Build history of the part. All positions in model axes, mm. A direction names the side the tool comes from. Give positions to 0.01 mm unless a question says otherwise; leave off trailing zeros. Order: outer loops, then holes, each group sorted by start corner. A loop starts at its lowest first (then second) coordinate and runs counter-clockwise, first axis right, second up. Notation, with made-up numbers: (59.25, 11.25) - (106.25, 11.25) arc R19 cw to (106.25, 41.25) - close; hole circle Ø10 at (23.5, -28). An arc over 180 degrees is marked (long way). Use a Markdown table: item, result. Add a question column.
(1) Flat gauge pins, fed straight in: pin 1 (2 mm diameter, centred on x = 8, z = 14, fed in from -Y); pin 2 (1.1 mm diameter, centred on y = -8.5, z = 4.5, fed in from +X); pin 3 (8 mm diameter, centred on x = 2, y = 4.5, fed in from +Z). Where does each tip first touch, or does it go through?
(2) Slice it at C-C (z = 12.5). Write the cut outline in (x, y).
(3) Slice it at B-B (y = 12). Write the cut outline in (x, z).
(4) Slice it at D-D (z = 21.5). Write the cut outline in (x, y).
(5) Wall check: line 1 (X direction, y = 4, z = 12.25); line 2 (Y direction, x = 0, z = 16.5); line 3 (Y direction, x = 0, z = 23.2). Give the ranges that are in metal, low to high.
(6) Which spindle directions (+Z, -Z, +X, -X, +Y, -Y) get a long thin tool onto all of the face, cutting with end or side? Do faces 5 (the face through (-2.17, -9.76, 19.96)), 6 (the face through (4.38, -8.43, 23.25)), 7 (the face through (6.3, -9, 7)), 8 (the face through (-8.8, -4.2, 7.4)). Say none if no direction does.
(7) Slice it at A-A (x = 0). Write the cut outline in (y, z).
(8) Mould opens along Z. For faces 1 (the face through (0, 13.5, 7)), 2 (the face through (0, 7, 15)), 3 (the face through (0, 13, 17)), 4 (the face through (9, -4, 23)) say: +Z half, -Z half, draft (parallel to the pull), parting line (faces both ways), or undercut.
from build123d import *

# Parameters (mm, degrees)
F1_DEPTH = 15
F3_DEPTH = 2
F4_R     = 11.5
F4_R_2   = 10
F5_DEPTH = 7
F6_R     = 11.5
F6_R_2   = 9.5
F7_DEPTH = 1
F8_R     = 0.5


with BuildPart() as f1:
    # F0 (on Top) → F1 (new body)
    with BuildSketch(Plane.XY):
        with BuildLine():
            ThreePointArc((-6.3, -7.4412700529), (-8.8455497285, -4.1010669343), (-9.75, 0))
            Line((-9.75, 0), (-11.5, 0))
            ThreePointArc((-11.5, 0), (-10.1168176815, -5.4680892458), (-6.3, -9.6208107766))
            Line((-6.3, -9.6208107766), (-6.3, -7.4412700529))
        make_face()
        with BuildLine():
            Line((11.5, 0), (9.75, 0))
            ThreePointArc((9.75, 0), (8.8455497285, -4.1010669343), (6.3, -7.4412700529))
            Line((6.3, -7.4412700529), (6.3, -9.6208107766))
            ThreePointArc((6.3, -9.6208107766), (10.1168176815, -5.4680892458), (11.5, 0))
        make_face()
        with BuildLine():
            Line((9.75, 13.5), (9.75, 6.0981554588))
            ThreePointArc((9.75, 6.0981554588), (11.0538454847, 3.1721443851), (11.5, 0))
            Line((11.5, 0), (11.5, 13.5))
            Line((11.5, 13.5), (9.75, 13.5))
        make_face()
        with BuildLine():
            Line((9.75, 6.0981554588), (9.75, 0))
            Line((9.75, 0), (11.5, 0))
            ThreePointArc((11.5, 0), (11.0538454847, 3.1721443851), (9.75, 6.0981554588))
        make_face()
        with BuildLine():
            ThreePointArc((-11.5, 0), (-11.0538454847, 3.1721443851), (-9.75, 6.0981554588))
            Line((-9.75, 6.0981554588), (-9.75, 13.5))
            Line((-9.75, 13.5), (-11.5, 13.5))
            Line((-11.5, 13.5), (-11.5, 0))
        make_face()
        with BuildLine():
            Line((-11.5, 0), (-9.75, 0))
            Line((-9.75, 0), (-9.75, 6.0981554588))
            ThreePointArc((-9.75, 6.0981554588), (-11.0538454847, 3.1721443851), (-11.5, 0))
        make_face()
        Polygon((-9.75, 13.5), (9.75, 13.5), (11.5, 13.5), (11.5, 15.583621338), (-11.5, 15.583621338), (-11.5, 13.5), align=None)
    extrude(amount=F1_DEPTH)

    # F2 (on face) → F3 (join)
    with BuildSketch(Plane.XY.offset(15)):
        with BuildLine():
            Line((11.5, 15.583621338), (-11.5, 15.583621338))
            Line((-11.5, 15.583621338), (-11.5, 0))
            ThreePointArc((-11.5, 0), (0, 11.5), (11.5, 0))
            Line((11.5, 0), (11.5, 15.583621338))
        make_face()
        with BuildLine():
            ThreePointArc((11.5, 0), (0, 11.5), (-11.5, 0))
            Line((-11.5, 0), (-6.25, 0))
            ThreePointArc((-6.25, 0), (0, 6.25), (6.25, 0))
            Line((6.25, 0), (11.5, 0))
        make_face()
        with BuildLine():
            Line((-6.25, 0), (-11.5, 0))
            ThreePointArc((-11.5, 0), (0, -11.5), (11.5, 0))
            Line((11.5, 0), (6.25, 0))
            ThreePointArc((6.25, 0), (0, -6.25), (-6.25, 0))
        make_face()
    extrude(amount=F3_DEPTH)

    # F4 (on face) → F5 (join)
    with BuildSketch(Plane.XY.offset(17)):
        Circle(F4_R)
        Circle(F4_R_2, mode=Mode.SUBTRACT)
    extrude(amount=F5_DEPTH)

    # F6 (on face) → F7 (join)
    with BuildSketch(Plane.XY.offset(24)):
        Circle(F6_R)
        Circle(F6_R_2, mode=Mode.SUBTRACT)
    extrude(amount=-F7_DEPTH)

    # F8
    f8_edges = [f1.edges().sort_by_distance(p)[0] for p in [
        (-9.5, 0, 24),
    ]]
    fillet(f8_edges, radius=F8_R)


solid = f1.part
Solution:
| question | item | result |
|---|---|---|
| 1 | pin 1 | y = -9.12 |
| 1 | pin 2 | x = 8.31 |
| 1 | pin 3 | z = 17 |
| 2 | outline | (-11.5, 0) arc R11.5 ccw to (-6.3, -9.62) - (-6.3, -7.44) arc R9.75 cw to (-9.75, 0) - (-9.75, 13.5) - (9.75, 13.5) - (9.75, 0) arc R9.75 cw to (6.3, -7.44) - (6.3, -9.62) arc R11.5 ccw to (11.5, 0) - (11.5, 15.58) - (-11.5, 15.58) - close |
| 3 | outline | (-11.5, 0) - (-9.75, 0) - (-9.75, 15) - (9.75, 15) - (9.75, 0) - (11.5, 0) - (11.5, 17) - (-11.5, 17) - close |
| 4 | outline | circle Ø23 at (0, 0); hole circle Ø20 at (0, 0) |
| 5 | line 1 | -11.5 to -9.75, 9.75 to 11.5 |
| 5 | line 2 | -11.5 to -6.25, 6.25 to 15.58 |
| 5 | line 3 | -11.5 to -9.5, 9.5 to 11.5 |
| 6 | face 5 | none |
| 6 | face 6 | +Z |
| 6 | face 7 | -Z, -Y |
| 6 | face 8 | -Z |
| 7 | outline | (-11.5, 15) - (-6.25, 15) - (-6.25, 17) - (-10, 17) - (-10, 23) - (-9.5, 23) - (-9.5, 23.5) arc R0.5 ccw to (-10, 24) - (-11.5, 24) - close; (6.25, 15) - (13.5, 15) - (13.5, 0) - (15.58, 0) - (15.58, 17) - (11.5, 17) - (11.5, 24) - (10, 24) arc R0.5 ccw to (9.5, 23.5) - (9.5, 23) - (10, 23) - (10, 17) - (6.25, 17) - close |
| 8 | face 1 | draft |
| 8 | face 2 | -Z half |
| 8 | face 3 | +Z half |
| 8 | face 4 | undercut |
